Verification items for the finished model (mm, model axes). Face numbers are marked on the shaded views. A direction names the side the tool comes from. Coordinates: 2 decimals unless noted, no trailing zeros. Order: outer loops, then holes, each group sorted by start corner. A loop starts at its lowest first (then second) coordinate and runs counter-clockwise, first axis right, second up. Notation, with made-up numbers: M 60.25,24 L 74.25,24 A19 ccw 74.25,58 Z; hole C 27.25,73.5 d7. An arc over 180 degrees is marked long. Return JSON: item names as keys, results as strings. Group by question number.
Q1. Section check B-B, the plane y = 10.5. Enter the section's corners in (x, z).
Q2. Thickness scan on probe 1 along Z at (x, y) = (-2.5, 11.75); probe 2 along X at (y, z) = (11, -0.5); probe 3 along Y at (x, z) = (11, 0). Record the ranges inside material, lowest first.
Q3. Mould release check, pull along Z, two halves, no side actions. Record for the marked faces 1, 2 and 3: pulls with the +Z half, pulls with the -Z half, needs draft (parallel to the pull), parting line crosses it, or undercut.
Q4. Access from +Z, -Z, +X, -X, +Y, -Y to the whole of each face (thin tool, end or side, straight path). Record for the marked faces 4, 5 and 6.
Q5. Section check D-D, the plane z = 5. Enter the section's corners in (x, y).
Q6. Go/stop test with flat-tipped pins: pin 1 Ø3.5 at (x, z) = (16.5, 0) entering from -Y; pin 2 Ø0.8 at (x, y) = (-9.5, 7.5) entering from +Z. Record where each tip stops, or that it passes through.
Q7. Section check A-A, the plane x = -10. Enter the section's corners in (y, z).
Q8. Section check C-C, the plane z = 8.75. Enter the section's corners in (x, y).
from build123d import *

# Parameters (mm, degrees)
SKETCH1_W           = 36
SKETCH1_H           = 21
BOSS_EXTRUDE2_DEPTH = 15
CUT_EXTRUDE1_DEPTH  = 15
SKETCH5_W           = 30
SKETCH5_H           = 15
CUT_EXTRUDE2_DEPTH  = 3.5
SKETCH7_W           = 30
SKETCH7_H           = 15
CUT_EXTRUDE3_DEPTH  = 5.5
FILLET1_R           = 1
FILLET2_R           = 1
SKETCH9_W           = 3
SKETCH9_H           = 3
BOSS_EXTRUDE3_DEPTH = 1
SKETCH9_4_W         = 3
SKETCH9_4_H         = 3
BOSS_EXTRUDE4_DEPTH = 1
SKETCH10_W          = 3
SKETCH10_H          = 1.5
BOSS_EXTRUDE5_DEPTH = 1
CUT_EXTRUDE4_DEPTH  = 35.296501279
SKETCH12_W          = 3
SKETCH12_H          = 6
BOSS_EXTRUDE6_DEPTH = 0.5
FILLET3_R           = 11
FILLET4_R           = 0.5
SKETCH17_W          = 3
SKETCH17_H          = 2
BOSS_EXTRUDE7_DEPTH = 1
SKETCH18_W          = 3
SKETCH18_H          = 1.5
BOSS_EXTRUDE8_DEPTH = 1
FILLET5_R           = 0.75
FILLET6_START       = -1.5
FILLET6_DEPTH       = 3
SKETCH19_W          = 3
SKETCH19_H          = 1
CUT_EXTRUDE5_DEPTH  = 8
SKETCH20_W          = 3
SKETCH20_H          = 2.565888667
CUT_EXTRUDE6_DEPTH  = 8
SKETCH21_W          = 4
SKETCH21_H          = 3
CUT_EXTRUDE7_DEPTH  = 8


with BuildPart() as part:
    # Sketch1 → Boss-Extrude2 (new body)
    with BuildSketch(Plane(origin=(0, 0, 0), x_dir=(1, 0, 0), z_dir=(0, 1, 0))):
        Rectangle(SKETCH1_W, SKETCH1_H)
    extrude(amount=BOSS_EXTRUDE2_DEPTH)

    # Sketch2 → Cut-Extrude1 (cut)
    with BuildSketch(Plane(origin=(18, 0, 0), x_dir=(0, 0, -1), z_dir=(1, 0, 0))):
        with BuildLine():
            Line((-4.2, 7.8), (4.2, 7.8))
            ThreePointArc((4.2, 7.8), (5.5, 6.5), (4.2, 5.2))
            Line((4.2, 5.2), (-4.2, 5.2))
            ThreePointArc((-4.2, 5.2), (-5.5, 6.5), (-4.2, 7.8))
        make_face()
    extrude(amount=-CUT_EXTRUDE1_DEPTH, mode=Mode.SUBTRACT)


with BuildPart() as body_2:
    # Split1: the piece on the far side of the plane
    add(part.part)
    split(bisect_by=Plane.ZX.offset(6.5), keep=Keep.BOTTOM)

    # Sketch5 → Cut-Extrude2 (cut)
    with BuildSketch(Plane(origin=(0, 6.5, 0), x_dir=(1, 0, 0), z_dir=(0, 1, 0))):
        Rectangle(SKETCH5_W, SKETCH5_H)
    extrude(amount=-CUT_EXTRUDE2_DEPTH, mode=Mode.SUBTRACT)

    # Fillet2
    fillet2_edges = [body_2.edges().sort_by_distance(p)[0] for p in [
        (18, 0, 0),
        (0, 0, -10.5),
        (-18, 0, 0),
        (0, 0, 10.5),
        (18, 3.25, 10.5),
        (-18, 3.25, 10.5),
        (-18, 3.25, -10.5),
        (18, 3.25, -10.5),
    ]]
    fillet(fillet2_edges, radius=FILLET2_R)

    # Sketch9 → Boss-Extrude3 (add)
    with BuildSketch(Plane.XY.offset(10.5)):
        with Locations((-9.5, 8)):
            Rectangle(SKETCH9_W, SKETCH9_H)
    extrude(amount=-BOSS_EXTRUDE3_DEPTH)

    # Sketch9<4> → Boss-Extrude4 (add)
    with BuildSketch(Plane.XY.offset(10.5)):
        with Locations((9.5, 8)):
            Rectangle(SKETCH9_4_W, SKETCH9_4_H)
    extrude(amount=-BOSS_EXTRUDE4_DEPTH)

    # Sketch10 → Boss-Extrude5 (add)
    with BuildSketch(Plane(origin=(0, 0, 9.5), x_dir=(-1, 0, 0), z_dir=(0, 0, -1))):
        with Locations((-9.5, 8.75)):
            Rectangle(SKETCH10_W, SKETCH10_H)
        with Locations((9.5, 8.75)):
            Rectangle(SKETCH10_W, SKETCH10_H)
    extrude(amount=BOSS_EXTRUDE5_DEPTH)

    # Sketch11 → Cut-Extrude4 (cut, through all)
    with BuildSketch(Plane(origin=(11, 0, 0), x_dir=(0, 0, -1), z_dir=(1, 0, 0))):
        Polygon((-9.5, 9.5), (-8.5, 8), (-8.5, 9.5), align=None)
    extrude(amount=-CUT_EXTRUDE4_DEPTH, mode=Mode.SUBTRACT)

    # Sketch12 → Boss-Extrude6 (add, symmetric)
    with BuildSketch(Plane(origin=(0, 0, -10.5), x_dir=(-1, 0, 0), z_dir=(0, 0, -1))):
        with Locations((0, 6.5)):
            Rectangle(SKETCH12_W, SKETCH12_H)
    extrude(amount=BOSS_EXTRUDE6_DEPTH, both=True)

    # Fillet3
    # the kernel refuses this fillet: 11 mm, written as the material it takes off along each edge
    with BuildSketch(Plane(origin=(-9.696798155, 3.5, -11), x_dir=(0, 0, 1), z_dir=(1, 0, 0))) as fillet3_piece_1:
        with BuildLine():
            CenterArc((11, -3.278719262), FILLET3_R, 162.658557197, 17.341442803)
            Line((0, -3.278719262), (-0.22, -3.278719262))
            Line((-0.22, -3.278719262), (-0.22, 0))
            Line((-0.22, 0), (0, 0.22))
            ThreePointArc((0, 0.22), (0.25, 0.22), (0.29, 0.065574385))
            Line((0.29, 0.065574385), (0.5, 0))
        make_face()
    extrude(amount=19.393596311, mode=Mode.SUBTRACT)

    # Fillet4
    fillet4_edges = [body_2.edges().sort_by_distance(p)[0] for p in [
        (-9.5, 9.5, 9.5),
        (9.5, 9.5, 9.5),
        (-9.5, 9.5, 10.5),
        (9.5, 9.5, 10.5),
    ]]
    fillet(fillet4_edges, radius=FILLET4_R)

    # Sketch17 → Boss-Extrude7 (add)
    with BuildSketch(Plane.XY.offset(-10)):
        with Locations((0, 10.5)):
            Rectangle(SKETCH17_W, SKETCH17_H)
    extrude(amount=-BOSS_EXTRUDE7_DEPTH)

    # Sketch18 → Boss-Extrude8 (add)
    with BuildSketch(Plane.XY.offset(-10)):
        with Locations((0, 9.25)):
            Rectangle(SKETCH18_W, SKETCH18_H)
    extrude(amount=BOSS_EXTRUDE8_DEPTH)

    # Fillet5
    fillet5_edges = [body_2.edges().sort_by_distance(p)[0] for p in [
        (0, 8.5, -9),
        (0, 10, -9),
    ]]
    fillet(fillet5_edges, radius=FILLET5_R - 0.0001)  # a hair under: the kernel refuses the full size

    # Fillet6: read off the stored shape, not the designer's step
    # Fillet6 outline → Fillet6 (cut)
    with BuildSketch(Plane.YZ.offset(FILLET6_START)):
        with BuildLine():
            add(Edge.make_bspline(
                [(11.5, -11), (11.5, -10), (10.5, -10)],
                knots=[0, 0, 0, 1, 1, 1], degree=2, weights=[1, 0.070710678, 1]))
            Line((11.5, -11), (11.5, -10))
            Line((11.5, -10), (10.5, -10))
        make_face()
    extrude(amount=FILLET6_DEPTH, mode=Mode.SUBTRACT)


with BuildPart() as part_1:
    add(part.part)

    # Split1
    split(bisect_by=Plane.ZX.offset(6.5), keep=Keep.TOP)

    # Sketch7 → Cut-Extrude3 (cut)
    with BuildSketch(Plane.XZ.offset(-6.5)):
        Rectangle(SKETCH7_W, SKETCH7_H)
    extrude(amount=-CUT_EXTRUDE3_DEPTH, mode=Mode.SUBTRACT)

    # Fillet1
    fillet1_edges = [part_1.edges().sort_by_distance(p)[0] for p in [
        (-18, 15, 0),
        (0, 15, 10.5),
        (18, 15, 0),
        (18, 10.75, 10.5),
        (-18, 10.75, 10.5),
        (-18, 10.75, -10.5),
        (18, 10.75, -10.5),
        (0, 15, -10.5),
    ]]
    fillet(fillet1_edges, radius=FILLET1_R)

    # Combine1: cut body 2
    add(body_2.part, mode=Mode.SUBTRACT)

    # Sketch19 → Cut-Extrude5 (cut)
    with BuildSketch(Plane.XY.offset(10.5)):
        with Locations((9.5, 8.5)):
            Rectangle(SKETCH19_W, SKETCH19_H)
        with Locations((-9.5, 8.5)):
            Rectangle(SKETCH19_W, SKETCH19_H)
    extrude(amount=-CUT_EXTRUDE5_DEPTH, mode=Mode.SUBTRACT)

    # Sketch20 → Cut-Extrude6 (cut)
    with BuildSketch(Plane(origin=(0, 0, -10.5), x_dir=(-1, 0, 0), z_dir=(0, 0, -1))):
        with Locations((0, 9.782944334)):
            Rectangle(SKETCH20_W, SKETCH20_H)
    extrude(amount=-CUT_EXTRUDE6_DEPTH, mode=Mode.SUBTRACT)

    # Sketch21 → Cut-Extrude7 (cut)
    with BuildSketch(Plane(origin=(18, 0, 0), x_dir=(0, 0, -1), z_dir=(1, 0, 0))):
        with Locations((-5.5, 10.5)):
            Rectangle(SKETCH21_W, SKETCH21_H)
    extrude(amount=-CUT_EXTRUDE7_DEPTH, mode=Mode.SUBTRACT)


solid = part_1.part
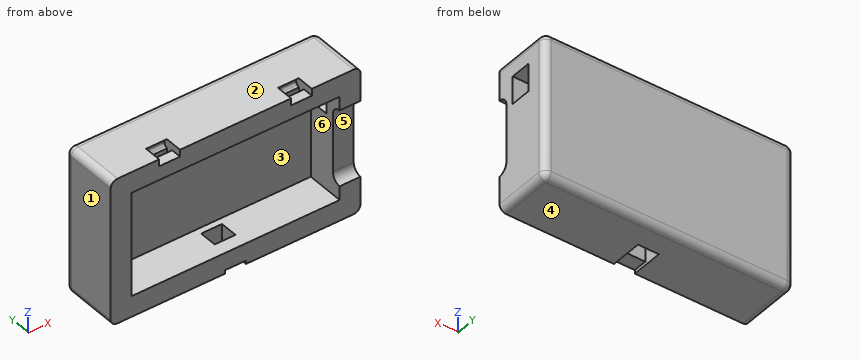
Numbers:
{
 "1": {"outline": "M -18,-9.5 A1 ccw -17,-10.5 L -1.5,-10.5 L -1.5,-7.5 L -15,-7.5 L -15,7.5 L 18,7.5 L 18,9.5 A1 ccw 17,10.5 L -17,10.5 A1 ccw -18,9.5 Z; M 1.5,-10.5 L 17,-10.5 A1 ccw 18,-9.5 L 18,3.5 L 15,3.5 L 15,-7.5 L 1.5,-7.5 Z"},
 "2": {"probe 1": "z = -10.5 to -7.5, 7.5 to 10.5", "probe 2": "x = -18 to -15, 15 to 18", "probe 3": "y = 12 to 15"},
 "3": {"face 1": "needs draft", "face 2": "pulls with the +Z half", "face 3": "undercut"},
 "4": {"face 4": "-Z, +X, -X, +Y, -Y", "face 5": "+X, -Y", "face 6": "-Y"},
 "5": {"outline": "M -18,6.5 L -15,6.5 L -15,12 L 18,12 L 18,14 A1 ccw 17,15 L -17,15 A1 ccw -18,14 Z; M 15,7.52 L 18,7.52 L 18,9 L 15,9 Z"},
 "6": {"pin 1": "stops at y = 7.8", "pin 2": "stops at z = 9.5"},
 "7": {"outline": "M 6.5,-10.5 L 14,-10.5 A1 ccw 15,-9.5 L 15,9.5 A1 ccw 14,10.5 L 9,10.5 A0.5 cw 9.5,10 L 9.5,9.77 A0.5 cw 9.28,9.35 L 9,9.17 L 9,7.5 L 12,7.5 L 12,-7.5 L 6.5,-7.5 Z; M 6.5,7.5 L 8,7.5 L 8,9.5 L 6.5,9.5 Z"},
 "8": {"outline": "M -18,6.5 L 18,6.5 L 18,14 A1 ccw 17,15 L -17,15 A1 ccw -18,14 Z; hole M -11,8 L -8,8 L -8,9 L -11,9 Z; hole M 8,8 L 11,8 L 11,9 L 8,9 Z"}
}
